```python
from build123d import *

# Parameters (mm, degrees)
BOSS_EXTRUDE1_DEPTH = 2
SKETCH2_W           = 18
SKETCH2_H           = 21
BOSS_EXTRUDE2_DEPTH = 11
SKETCH3_W           = 18
SKETCH3_H           = 21
BOSS_EXTRUDE3_DEPTH = 18.5
SKETCH4_W           = 12.5
SKETCH4_H           = 5
BOSS_EXTRUDE4_DEPTH = 11


with BuildPart() as part:
    # Sketch1 → Boss-Extrude1 (new body)
    with BuildSketch(Plane(origin=(0, 0, 0), x_dir=(1, 0, 0), z_dir=(0, 1, 0))):
        Polygon((-1, 12.75), (-20, 12.75), (-25, 7.75), (-25, -19.25), (25, -19.25), (25, 15.25), (21, 19.25), (5.5, 19.25), align=None)
    extrude(amount=BOSS_EXTRUDE1_DEPTH)

    # Sketch2 → Boss-Extrude2 (add)
    with BuildSketch(Plane(origin=(0, 2, 0), x_dir=(1, 0, 0), z_dir=(0, 1, 0))):
        with Locations((-10, -4.75)):
            Rectangle(SKETCH2_W, SKETCH2_H)
    extrude(amount=BOSS_EXTRUDE2_DEPTH)

    # Sketch3 → Boss-Extrude3 (add)
    with BuildSketch(Plane(origin=(0, 2, 0), x_dir=(1, 0, 0), z_dir=(0, 1, 0))):
        with Locations((11.471056506, -4.75)):
            Rectangle(SKETCH3_W, SKETCH3_H)
    extrude(amount=BOSS_EXTRUDE3_DEPTH)

    # Sketch4 → Boss-Extrude4 (add)
    with BuildSketch(Plane(origin=(0, 2, 0), x_dir=(1, 0, 0), z_dir=(0, 1, 0))):
        with Locations((14.75, 12.75)):
            Rectangle(SKETCH4_W, SKETCH4_H)
    extrude(amount=BOSS_EXTRUDE4_DEPTH)


solid = part.part
```
CAD build for the part. Positions are in the model's coordinates, mm. A direction names the side the tool comes from. Round coordinates to 2 decimals unless told otherwise and drop trailing zeros. Order: outer loops, then holes, each group sorted by start corner. A loop starts at its lowest first (then second) coordinate and runs counter-clockwise, first axis right, second up. Notation, with made-up numbers: (46.25, -6) - (93.25, -6) arc R8 ccw to (93.25, 6) - close; hole circle Ø8 at (88.5, -23). An arc over 180 degrees is marked (long way). Answer in a Markdown table with one row per item. Add a question column.
(1) Band-saw the part on B-B on x = -2.5. List the corners of the cut face in (y, z).
(2) Drop flat-ended pins along their axis: pin 1 Ø5.5 at (x, y) = (-10.5, 7.5) entering from -Z; pin 2 Ø0.6 at (x, y) = (-13, 1.5) entering from -Z; pin 3 Ø10 at (x, y) = (-19, 16) entering from +Z; pin 4 Ø1 at (y, z) = (8, -8) entering from -X. Give the stop position or say it passes through.
(3) Band-saw the part on C-C on z = -12. List the corners of the cut face in (x, y).
(4) Band-saw the part on A-A on y = 9.75. List the corners of the cut face in (x, z).
(5) Probe L1, parallel to Z at x = 15, y = 8; L2, parallel to X at y = 10.25, z = 11.5; L3, parallel to Y at x = -3, z = 1.5. List the from-to ranges inside material, lowest first. Write a range as [from, to].
(6) 3-axis set-ups, long thin cutter, end or side, ignore diameter. For faces 1 (the face through (21, 7, -13)), 2 (the face through (15, 7, -10.25)), 3 (the face through (15, 7, -15.25)), 4 (the face through (-10, 7, 15.25)): which of +Z, -Z, +X, -X, +Y, -Y reach the whole face in a straight line?
(7) Band-saw the part on D-D on x = 13. List the corners of the cut face in (y, z), and give its area (4 significant figures).
Data:
| question | item | result |
|---|---|---|
| 1 | outline | (0, -12.75) - (2, -12.75) - (2, -5.75) - (13, -5.75) - (13, 15.25) - (2, 15.25) - (2, 19.25) - (0, 19.25) - close |
| 2 | pin 1 | stops at z = -5.75 |
| 2 | pin 2 | stops at z = -12.75 |
| 2 | pin 3 | stops at z = 15.25 |
| 2 | pin 4 | passes through |
| 3 | outline | (-20.75, 0) - (25, 0) - (25, 2) - (21, 2) - (21, 13) - (8.5, 13) - (8.5, 2) - (-20.75, 2) - close |
| 4 | outline | (-19, -5.75) - (-1, -5.75) - (-1, 15.25) - (-19, 15.25) - close; (2.47, -5.75) - (20.47, -5.75) - (20.47, 15.25) - (2.47, 15.25) - close; (8.5, -15.25) - (21, -15.25) - (21, -10.25) - (8.5, -10.25) - close |
| 5 | L1 | z = [-15.25, -10.25], [-5.75, 15.25] |
| 5 | L2 | x = [-19, -1], [2.47, 20.47] |
| 5 | L3 | y = [0, 13] |
| 6 | face 1 | +Z, -Z, +X, +Y |
| 6 | face 2 | +X, -X, +Y |
| 6 | face 3 | -Z, +X, -X, +Y |
| 6 | face 4 | +Z, +X, -X, +Y |
| 7 | outline | (0, -19.25) - (2, -19.25) - (2, -15.25) - (13, -15.25) - (13, -10.25) - (2, -10.25) - (2, -5.75) - (20.5, -5.75) - (20.5, 15.25) - (2, 15.25) - (2, 19.25) - (0, 19.25) - close |
| 7 | area | 520.5 mm^2 |
